Model file for the job. Use its own axes, mm. Face numbers are marked on the shaded views. A direction names the side the tool comes from. Round coordinates to 2 decimals unless told otherwise and drop trailing zeros. Order: outer loops, then holes, each group sorted by start corner. A loop starts at its lowest first (then second) coordinate and runs counter-clockwise, first axis right, second up. Notation, with made-up numbers: (75, 74.25) - (114, 74.25) arc R27 cw to (114, 113.25) - close; hole circle Ø1 at (8.25, 67.25). An arc over 180 degrees is marked (long way). Write item = value, one per line.
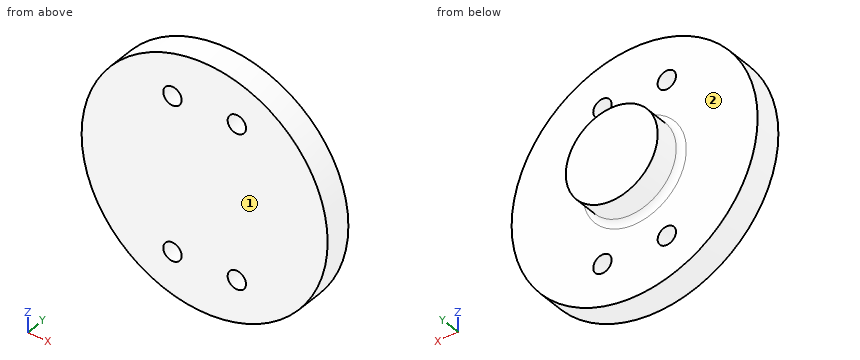
```python
from build123d import *

# Parameters (mm, degrees)
CROQUIS1_R              = 85
SALIENTE_EXTRUIR1_DEPTH = 19.05
CROQUIS2_R              = 31.75
SALIENTE_EXTRUIR2_DEPTH = 21
REDONDEO1_R             = 4
CROQUIS3_R              = 6.35
CORTAR_EXTRUIR1_DEPTH   = 19.05


with BuildPart() as part:
    # Croquis1 → Saliente-Extruir1 (new body)
    with BuildSketch(Plane(origin=(0, 0, 0), x_dir=(1, 0, 0), z_dir=(0, 1, 0))):
        Circle(CROQUIS1_R)
    extrude(amount=SALIENTE_EXTRUIR1_DEPTH)

    # Croquis2 → Saliente-Extruir2 (add)
    with BuildSketch(Plane(origin=(0, 19.05, 0), x_dir=(1, 0, 0), z_dir=(0, 1, 0))):
        Circle(CROQUIS2_R)
    extrude(amount=SALIENTE_EXTRUIR2_DEPTH)

    # Redondeo1
    redondeo1_edges = [part.edges().sort_by_distance(p)[0] for p in [
        (-31.75, 19.05, 0),
    ]]
    fillet(redondeo1_edges, radius=REDONDEO1_R)

    # Croquis3 → Cortar-Extruir1 (cut)
    with BuildSketch(Plane(origin=(0, 19.05, 0), x_dir=(1, 0, 0), z_dir=(0, 1, 0))):
        with Locations((-22.25, -53)):
            Circle(CROQUIS3_R)
        with Locations((-22.25, 53)):
            Circle(CROQUIS3_R)
        with Locations((22.25, 53)):
            Circle(CROQUIS3_R)
        with Locations((22.25, -53)):
            Circle(CROQUIS3_R)
    extrude(amount=-CORTAR_EXTRUIR1_DEPTH, mode=Mode.SUBTRACT)


solid = part.part
```
1) Cut at D-D (z = 53). Write the cut outline in (x, y), and give its area (3 significant figures).
Conclusion:
outline = (-66.45, 0) - (-28.6, 0) - (-28.6, 19.05) - (-66.45, 19.05) - close; (-15.9, 0) - (15.9, 0) - (15.9, 19.05) - (-15.9, 19.05) - close; (28.6, 0) - (66.45, 0) - (66.45, 19.05) - (28.6, 19.05) - close
area = 2,050 mm^2
2) Flat gauge pins, fed straight in: pin 1 Ø4 at (x, y) = (18.5, 29) entering from +Z; pin 2 Ø8 at (x, y) = (27, 5) entering from -Z; pin 3 Ø20.5 at (x, z) = (-22.25, 53) entering from +Y. Where does each tip first touch, or does it go through?
Conclusion:
pin_1 = 27.13
pin_2 = -81.83
pin_3 = 19.05
3) Wall check: line 1 along Z through (x, y) = (22.25, 11.25); line 2 along X through (y, z) = (5.5, 53.5); line 3 along X through (y, z) = (8.5, 53). Give the ranges that are in metal, low to high.
Conclusion:
line_1 = -82.04 to -59.35, -46.65 to 46.65, 59.35 to 82.04
line_2 = -66.05 to -28.58, -15.92 to 15.92, 28.58 to 66.05
line_3 = -66.45 to -28.6, -15.9 to 15.9, 28.6 to 66.45
4) Cut at A-A (z = 0). Write the cut outline in (x, y), and give its area (3 significant figures).
Conclusion:
outline = (-85, 0) - (85, 0) - (85, 19.05) - (35.75, 19.05) arc R4 cw to (31.75, 23.05) - (31.75, 40.05) - (-31.75, 40.05) - (-31.75, 23.05) arc R4 cw to (-35.75, 19.05) - (-85, 19.05) - close
area = 4,580 mm^2
5) Cut at B-B (y = 4). Write the cut outline in (x, z).
Conclusion:
outline = circle Ø170 at (0, 0); hole circle Ø12.7 at (-22.25, -53); hole circle Ø12.7 at (-22.25, 53); hole circle Ø12.7 at (22.25, -53); hole circle Ø12.7 at (22.25, 53)
6) Cut at C-C (x = 0). Write the cut outline in (y, z).
Conclusion:
outline = (0, -85) - (19.05, -85) - (19.05, -35.75) arc R4 cw to (23.05, -31.75) - (40.05, -31.75) - (40.05, 31.75) - (23.05, 31.75) arc R4 cw to (19.05, 35.75) - (19.05, 85) - (0, 85) - close
7) 3-axis set-ups, long thin cutter, end or side, ignore diameter. For the marked faces 1 and 2: which of +Z, -Z, +X, -X, +Y, -Y reach the whole face in a straight line?
Conclusion:
face_1 = +Z, -Z, +X, -X, -Y
face_2 = +Y
